```python
from build123d import *

# Parameters (mm, degrees)
F0_W     = 76.2
F0_H     = 76.2
F1_DEPTH = 76.2
F2_R     = 13.9945957695
F3_DEPTH = 76.2
F5_DEPTH = 76.2
F6_DEPTH = 0.127


# Not quite as in the source:
# - a feature of the source that left no trace in its solid (it failed there, or was rolled back) is left out


with BuildPart() as f1:
    # F0 (on Front) → F1 (new body)
    with BuildSketch(Plane.XZ):
        with Locations((-0.348880887, -0.3284779671)):
            Rectangle(F0_W, F0_H)
    extrude(amount=F1_DEPTH)

    # F2 (on face) → F3 (join)
    with BuildSketch(Plane(origin=(0, 0, 0), x_dir=(-1, 0, 0), z_dir=(0, 1, 0))):
        Circle(F2_R)
    extrude(amount=F3_DEPTH)

    # F4 (on face) → F5 (join)
    with BuildSketch(Plane(origin=(0, 0, 0), x_dir=(-1, 0, 0), z_dir=(0, 1, 0))):
        with BuildLine():
            ThreePointArc((12.5814202737, 6.1283419167), (21.0911235736, 6.5413963555), (25.2311478041, 13.9875942841))
            ThreePointArc((25.2311478041, 13.9875942841), (15.1695556684, 22.6577098126), (8.081240073, 11.4255096006))
            ThreePointArc((8.081240073, 11.4255096006), (10.6654291765, 9.0607577626), (12.5814202737, 6.1283419167))
        make_face()
        with BuildLine():
            ThreePointArc((13.1726915392, -4.7253474332), (11.363857458, -8.1677080277), (8.6776055388, -10.9794295328))
            ThreePointArc((8.6776055388, -10.9794295328), (16.220264771, -20.1665195025), (24.895431247, -12.0402770117))
            ThreePointArc((24.895431247, -12.0402770117), (21.0629315641, -5.1313910488), (13.1726915392, -4.7253474332))
        make_face()
        with BuildLine():
            ThreePointArc((13.1726915392, -4.7253474332), (10.1390684725, -7.2873978983), (8.6776055388, -10.9794295328))
            ThreePointArc((8.6776055388, -10.9794295328), (11.363857458, -8.1677080277), (13.1726915392, -4.7253474332))
        make_face()
    extrude(amount=F5_DEPTH)

    # F6 (add): a face of the model
    f6_faces = [f1.faces().sort_by_distance(p)[0] for p in [
        (-6.9646133447, 76.2, 0.8386205015),
    ]]
    extrude(f6_faces, amount=F6_DEPTH)


solid = f1.part
```
Here's how the part is built. I have some questions about the finished solid (model axes, mm). A direction names the side the tool comes from. Give positions to 0.01 mm unless a question says otherwise; leave off trailing zeros. Order: outer loops, then holes, each group sorted by start corner. A loop starts at its lowest first (then second) coordinate and runs counter-clockwise, first axis right, second up. Notation, with made-up numbers: M 49,57.5 L 92,57.5 A32 cw 92,91.5 Z; hole C 21,14.25 d3. An arc over 180 degrees is marked long. Use a Markdown table: item, result. Add a question column.
1. I need wall thicknesses on probe 1 along Y at (x, z) = (-22, 2.5); probe 2 along Z at (x, y) = (-18, 35.5); probe 3 along Z at (x, y) = (-18.5, 21.5). Which ranges of each line are inside material? Lowest first, please. Write a range as from..to.
2. Suppose I cut it at A-A (z = 0). List the corners of the cut face in (x, y) for me.
3. On a 3-axis mill with a long thin cutter (end or side, diameter ignored), from which of +Z, -Z, +X, -X, +Y, -Y can I reach the whole of each face in a straight line? I mean faces 1 (the flat face through (16, 0, 0)), 2 (the flat face through (-1, -38, 37.772)). Say none if no direction works.
4. Suppose I cut it at D-D (x = -29.5). List the corners of the cut face in (y, z) for me.
5. If we mould it in two halves opening along X, with no side actions, what happens to faces 3 (the flat face through (-38.449, -38, -1)), 4 (the cylindrical face through (13.994, 37.629, 0.061)), 5 (the flat face through (-5, 76.327, 2)), 6 (the cylindrical face through (-13.97, 37.63, 0.84))? For each: +X half, -X half, draft (parallel to the pull), parting line (faces both ways), or undercut.
6. Suppose I cut it at C-C (z = -27.5). List the corners of the cut face in (x, y) for me, and give its area (3 significant figures).
7. Suppose I cut it at B-B (x = 0). List the corners of the cut face in (y, z) for me.
8. For pin 1 Ø5 at (x, z) = (-4.5, -22.5) entering from +Y, with a flat end and sliding along its axis, tell me the tip position at first contact or that it passes through.
Results list:
| question | item | result |
|---|---|---|
| 1 | probe 1 | y = -76.2..0 |
| 1 | probe 2 | z = -20.09..-3.99, 5.36..22.62 |
| 1 | probe 3 | z = -19.99..-4.09, 5.46..22.51 |
| 2 | outline | M -38.45,-76.2 L 37.75,-76.2 L 37.75,0 L 13.99,0 L 13.99,76.33 L -13.99,76.33 L -13.99,0 L -38.45,0 Z |
| 3 | face 1 | +Y |
| 3 | face 2 | +Z, +X, -X, +Y, -Y |
| 4 | outline | M -76.2,-38.43 L 0,-38.43 L 0,37.77 L -76.2,37.77 Z |
| 5 | face 3 | -X half |
| 5 | face 4 | undercut |
| 5 | face 5 | draft |
| 5 | face 6 | undercut |
| 6 | outline | M -38.45,-76.2 L 37.75,-76.2 L 37.75,0 L -38.45,0 Z |
| 6 | area | 5,810 mm² |
| 7 | outline | M -76.2,-38.43 L 0,-38.43 L 0,-13.99 L 76.33,-13.99 L 76.33,13.99 L 0,13.99 L 0,37.77 L -76.2,37.77 Z |
| 8 | pin 1 | stops at y = 0 |
